from build123d import *

# Parameters (mm, degrees)
SKETCH1_R           = 37.5
SKETCH1_R_2         = 18
BOSS_EXTRUDE1_DEPTH = 5
SKETCH2_R           = 25
CUT_EXTRUDE1_DEPTH  = 3
SKETCH3_OUTSIDE_W   = 98.236
SKETCH3_OUTSIDE_H   = 98.236
SKETCH3_OUTSIDE_W_2 = 62
SKETCH3_OUTSIDE_H_2 = 62
CUT_EXTRUDE2_DEPTH  = 6
SKETCH4_R           = 2.75
CUT_EXTRUDE3_DEPTH  = 6


with BuildPart() as part:
    # Sketch1 → Boss-Extrude1 (new body)
    with BuildSketch(Plane(origin=(0, 0, 0), x_dir=(1, 0, 0), z_dir=(0, 1, 0))):
        Circle(SKETCH1_R)
        Circle(SKETCH1_R_2, mode=Mode.SUBTRACT)
    extrude(amount=BOSS_EXTRUDE1_DEPTH)

    # Sketch2 → Cut-Extrude1 (cut)
    with BuildSketch(Plane(origin=(0, 5, 0), x_dir=(1, 0, 0), z_dir=(0, 1, 0))):
        Circle(SKETCH2_R)
    extrude(amount=-CUT_EXTRUDE1_DEPTH, mode=Mode.SUBTRACT)

    # Sketch3 outside → Cut-Extrude2 (cut, through all)
    with BuildSketch(Plane(origin=(0, 5, 0), x_dir=(1, 0, 0), z_dir=(0, 1, 0))):
        Rectangle(SKETCH3_OUTSIDE_W, SKETCH3_OUTSIDE_H)
        Rectangle(SKETCH3_OUTSIDE_W_2, SKETCH3_OUTSIDE_H_2, mode=Mode.SUBTRACT)
    extrude(amount=-CUT_EXTRUDE2_DEPTH, mode=Mode.SUBTRACT)

    # Sketch4 → Cut-Extrude3 (cut, through all)
    with BuildSketch(Plane(origin=(0, 5, 0), x_dir=(1, 0, 0), z_dir=(0, 1, 0))):
        with Locations((-22.627416998, 22.627416998)):
            Circle(SKETCH4_R)
        with Locations((22.627416998, 22.627416998)):
            Circle(SKETCH4_R)
        with Locations((22.627416998, -22.627416998)):
            Circle(SKETCH4_R)
        with Locations((-22.627416998, -22.627416998)):
            Circle(SKETCH4_R)
    extrude(amount=-CUT_EXTRUDE3_DEPTH, mode=Mode.SUBTRACT)


solid = part.part
Work out the finished part from the listing and answer in its coordinate system (mm). A direction names the side the tool comes from. Coordinates: 2 decimals unless noted, no trailing zeros. Loops run counter-clockwise (first coordinate to the right, second up) from the corner with the lowest first, then second, coordinate; pieces in that order, holes last. Notation, with made-up numbers: (66.5, 23.5) -> (120.5, 23.5) arc R28 cw to (120.5, 56.5) -> close; hole circle Ø1 at (-22, -2). An arc over 180 degrees is marked (long way). Answer as CSV lines item,"result".
1) For faces 1 (the face through (11, 2, 16)), 2 (the face through (31, 3, 0)), determine the directions among +Z, -Z, +X, -X, +Y, -Y from which every point of the face is accessible in a straight line to the end or side of a thin tool.
A:
face 1,"+Y"
face 2,"+Z, -Z, +X, +Y, -Y"
2) For a pull along Z with two mould halves and no side action, classify faces 3 (the face through (26.447, 2.465, 26.586)), 4 (the face through (-21, 5, -14)), 5 (the face through (-22.99, 2.54, 19.9)) as released by +Z, released by -Z, zero draft, split by the parting line, or undercut.
A:
face 3,"released by +Z"
face 4,"zero draft"
face 5,"undercut"
3) Flat-ended cylindrical pins translate along their axes: pin 1 (1 mm diameter, centred on x = -22.5, y = 1.5, fed in from -Z); pin 2 (1 mm diameter, centred on x = -13.5, z = -14, fed in from +Y). Find the tip coordinate at first contact, or state that the pin passes through.
A:
pin 1,"stops at z = -30.37"
pin 2,"stops at y = 2"
4) The part is cut by section B-B (z = 0). Give the vertices of the cut face in (x, y).
A:
outline,"(-31, 0) -> (-18, 0) -> (-18, 2) -> (-25, 2) -> (-25, 5) -> (-31, 5) -> close; (18, 0) -> (31, 0) -> (31, 5) -> (25, 5) -> (25, 2) -> (18, 2) -> close"
5) Straight lines are drawn through the part: probe 1 along Z at (x, y) = (0, 1.15); probe 2 along Z at (x, y) = (0, 3.1). For each, find the intervals that lie inside material, in ascending order.
A:
probe 1,"z = -31 to -18, 18 to 31"
probe 2,"z = -31 to -25, 25 to 31"
6) The part is cut by section A-A (x = 0). Give the vertices of the cut face in (y, z).
A:
outline,"(0, -31) -> (5, -31) -> (5, -25) -> (2, -25) -> (2, -18) -> (0, -18) -> close; (0, 18) -> (2, 18) -> (2, 25) -> (5, 25) -> (5, 31) -> (0, 31) -> close"
